Geometry: see drawing. Coordinates: mm, zero at the bounding-box minimum. A direction names the side the tool comes from. Coordinates: 2 decimals unless noted, no trailing zeros. Write each loop counter-clockwise with the first axis right and the second up, starting at its lowest first coordinate (ties: lowest second). Pieces come first, ordered by that corner, then holes. Notation, with made-up numbers: (-2, -32.75) - (19, -32.75) arc R34 cw to (19, -1.75) - close; hole circle Ø7 at (60, 33.5). An arc over 180 degrees is marked (long way). One line per question, with ' | ' between items. Start each with the question number.
1) First-contact query: P1, Ø3.5, axis at y = 16.67, z = 7.8, coming from the -X side; P2, Ø3, axis at y = 9.5, z = 11, coming from the +X side; P3, Ø6.5, axis at x = 9, z = 7.5, coming from the +Y side. Flat tips, straight axial feed; report the tip coordinate or a pass-through.
2) Reachability of the marked faces 1, 2, 3 and 4 from +Z, -Z, +X, -X, +Y, -Y: full face, straight path, thin tool, end or side. Return the list, or none.
3) Line query: line 1 (Y direction, x = 23.45, z = 7.8); line 2 (X direction, y = 14, z = 3); line 3 (Y direction, x = 27.5, z = 8). Output: solid intervals per line, ascending.
4) Section query D-D on z = 10.7. Return loops of the section in (x, y).
5) Draft query along X for the marked faces 5, 6 and 7. Return one class per face: released by +X, released by -X, zero draft, split by the parting line, or undercut.
6) Section query C-C on y = 13.25. Return loops of the section in (x, z).
7) Section query B-B on z = 7.8. Return loops of the section in (x, y).
8) Section query A-A on x = 33.1. Return loops of the section in (y, z), and give its area (3 significant figures).
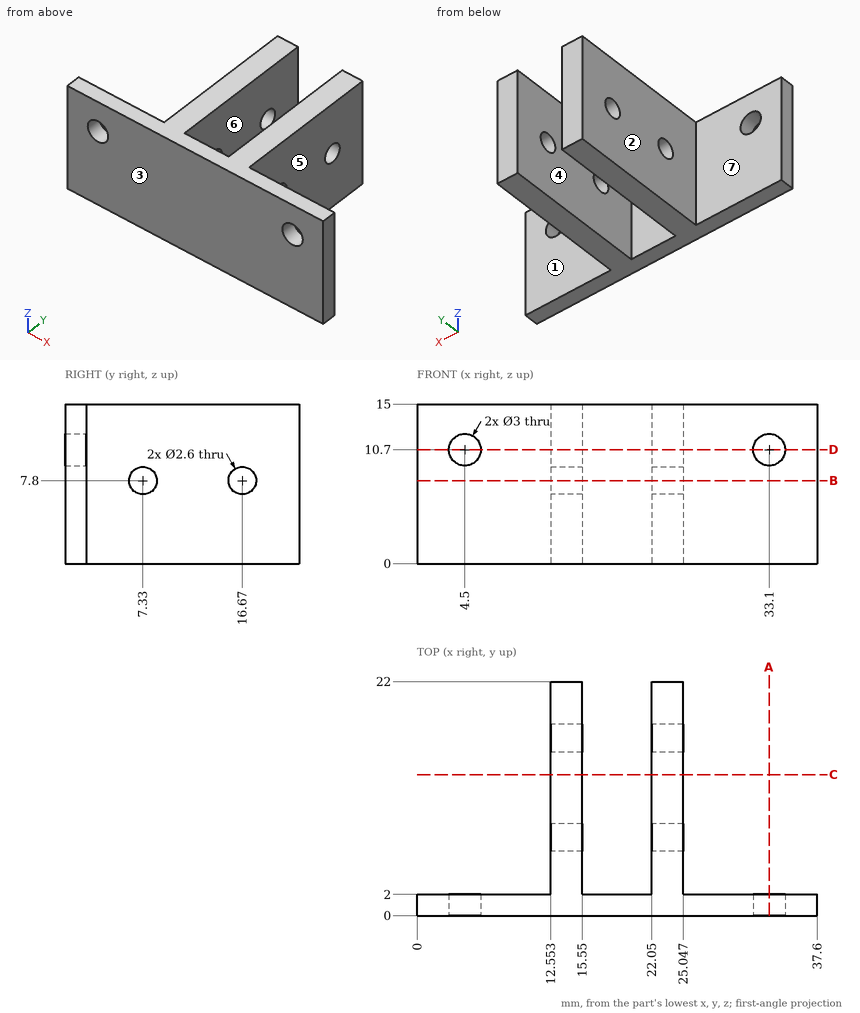
Answer key:
1) P1: x = 12.55 | P2: x = 25.05 | P3: y = 2
2) face 1: +Z, -Z, +X, +Y | face 2: +Z, -Z, -X, +Y | face 3: +Z, -Z, +X, -X, -Y | face 4: +Z, -Z, +Y
3) line 1: 0 to 6.03, 8.63 to 15.37, 17.97 to 22 | line 2: 12.55 to 15.55, 22.05 to 25.05 | line 3: 0 to 2
4) outline: (0, 0) - (3, 0) - (3, 2) - (0, 2) - close; (6, 0) - (31.6, 0) - (31.6, 2) - (25.05, 2) - (25.05, 22) - (22.05, 22) - (22.05, 2) - (15.55, 2) - (15.55, 22) - (12.55, 22) - (12.55, 2) - (6, 2) - close; (34.6, 0) - (37.6, 0) - (37.6, 2) - (34.6, 2) - close
5) face 5: released by +X | face 6: undercut | face 7: zero draft
6) outline: (12.55, 0) - (15.55, 0) - (15.55, 15) - (12.55, 15) - close; (22.05, 0) - (25.05, 0) - (25.05, 15) - (22.05, 15) - close
7) outline: (0, 0) - (37.6, 0) - (37.6, 2) - (25.05, 2) - (25.05, 6.03) - (22.05, 6.03) - (22.05, 2) - (15.55, 2) - (15.55, 6.03) - (12.55, 6.03) - (12.55, 2) - (0, 2) - close; (12.55, 8.63) - (15.55, 8.63) - (15.55, 15.37) - (12.55, 15.37) - close; (12.55, 17.97) - (15.55, 17.97) - (15.55, 22) - (12.55, 22) - close; (22.05, 8.63) - (25.05, 8.63) - (25.05, 15.37) - (22.05, 15.37) - close; (22.05, 17.97) - (25.05, 17.97) - (25.05, 22) - (22.05, 22) - close
8) outline: (0, 0) - (2, 0) - (2, 9.2) - (0, 9.2) - close; (0, 12.2) - (2, 12.2) - (2, 15) - (0, 15) - close | area: 24.0 mm²
